CAD build for the part. Positions are in the model's coordinates, mm. Face numbers are marked on the shaded views. Coordinates: 2 decimals unless noted, no trailing zeros. Loops run counter-clockwise (first coordinate to the right, second up) from the corner with the lowest first, then second, coordinate; pieces in that order, holes last. Notation, with made-up numbers: M 31,33 L 53,33 A13 cw 53,50 Z; hole C 39.5,-0.5 d1. An arc over 180 degrees is marked long. Answer as a JSON object with one key per item and string values. Group by question number.
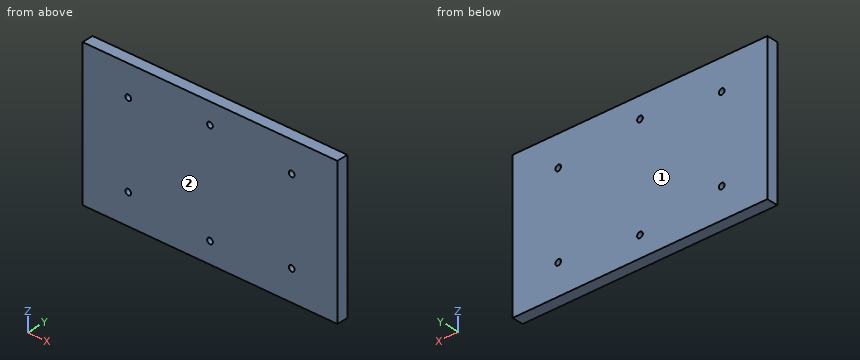
```python
from build123d import *

# Parameters (mm, degrees)
F0_W     = 425.45
F0_H     = 241.3
F1_DEPTH = 19.05
F2_D     = 9.525
F3_D     = 9.525
F4_D     = 9.525
F5_D     = 9.525
F6_D     = 9.525
F7_D     = 9.525


with BuildPart() as f1:
    # F0 (on Front) → F1 (new body)
    with BuildSketch(Plane.XZ):
        Rectangle(F0_W, F0_H)
    extrude(amount=F1_DEPTH)

    # F2 (through all)
    with Locations(Plane(origin=(0, 0, 0), x_dir=(1, 0, 0), z_dir=(0, 1, 0))):
        with Locations((136.525, 69.85)):
            Hole(F2_D / 2)

    # F3 (through all)
    with Locations(Plane(origin=(0, 0, 0), x_dir=(1, 0, 0), z_dir=(0, 1, 0))):
        with Locations((136.525, -69.85)):
            Hole(F3_D / 2)

    # F4 (through all)
    with Locations(Plane(origin=(0, 0, 0), x_dir=(1, 0, 0), z_dir=(0, 1, 0))):
        with Locations((-136.525, 69.85)):
            Hole(F4_D / 2)

    # F5 (through all)
    with Locations(Plane(origin=(0, 0, 0), x_dir=(1, 0, 0), z_dir=(0, 1, 0))):
        with Locations((-136.525, -69.85)):
            Hole(F5_D / 2)

    # F6 (through all)
    with Locations(Plane(origin=(0, 0, 0), x_dir=(1, 0, 0), z_dir=(0, 1, 0))):
        with Locations((0, 85.725)):
            Hole(F6_D / 2)

    # F7 (through all)
    with Locations(Plane(origin=(0, 0, 0), x_dir=(1, 0, 0), z_dir=(0, 1, 0))):
        with Locations((0, -85.725)):
            Hole(F7_D / 2)


solid = f1.part
```
Item 1: Slice it at A-A, the plane z = -69.85. Count the separate pieces of the cut face and the enclosed holes in it, then the cut area to 3 significant figures.
Item 2: Pin check, flat tip, straight feed: pin 1 (7.5 mm diameter, centred on x = 0, z = -85.725, fed in from +Y). Stop position of the tip, or through.
Item 3: Pull direction Y, two halves, no side cores. Call the marked faces 1 and 2: released by +Y, released by -Y, zero draft, split by the parting line, or undercut.
Item 4: Drill centre lines: L1, parallel to X at y = -13.75, z = 69.85 (1 decimal); L2, parallel to Z at x = 0, y = -14.25; L3, parallel to Z at x = -138, y = -2.25. Where is each one in solid material? Low to high. Write a range as from..to.
Item 5: Slice it at B-B, the plane x = 0. Write the cut outline in (y, z), then the cut area to 3 significant figures.
Computed:
{
 "1": {"separate pieces": "3", "enclosed holes": "0", "area": "7,740 mm2"},
 "2": {"pin 1": "through"},
 "3": {"face 1": "released by +Y", "face 2": "released by -Y"},
 "4": {"L1": "-212.7..-141.3, -131.8..131.8, 141.3..212.7", "L2": "-120.65..-90.49, -80.96..80.96, 90.49..120.65", "L3": "-120.65..-74.38, -65.32..65.32, 74.38..120.65"},
 "5": {"outline": "M -19.05,-120.65 L 0,-120.65 L 0,-90.49 L -19.05,-90.49 Z; M -19.05,-80.96 L 0,-80.96 L 0,80.96 L -19.05,80.96 Z; M -19.05,90.49 L 0,90.49 L 0,120.65 L -19.05,120.65 Z", "area": "4,230 mm2"}
}
